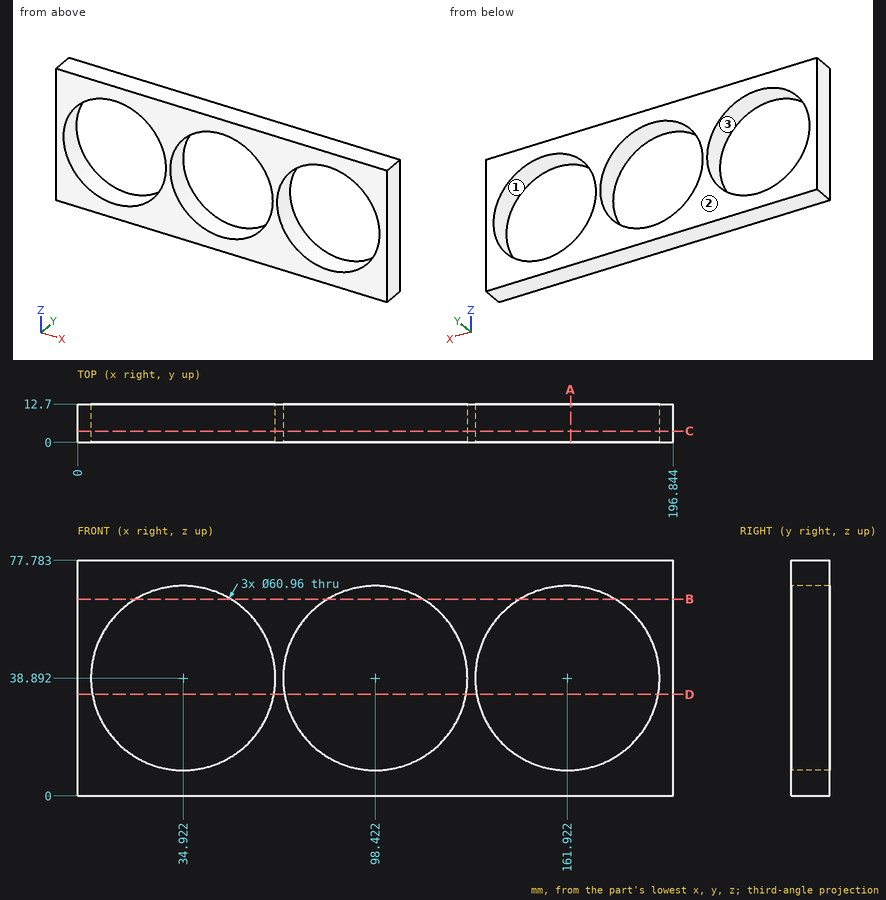
Answer from the drawing. Dimensions are ordinates in mm from the lowest x, y and z of the part. Give positions to 0.01 mm unless a question says otherwise; leave off trailing zeros. Write each loop counter-clockwise with the first axis right and the second up, starting at its lowest first coordinate (ties: lowest second). Pieces come first, ordered by that corner, then holes. Notation, with made-up numbers: M -5,53.5 L 49,53.5 A21 ccw 49,71.5 Z; hole C 56,36.25 d3. An arc over 180 degrees is marked long. Answer as CSV lines item,"result".
Q1. A cutting plane is placed at A-A on x = 163. Write down the section's boundary in (y, z), plus the area to 3 significant figures.
A:
outline,"M 0,0 L 12.7,0 L 12.7,8.43 L 0,8.43 Z; M 0,69.35 L 12.7,69.35 L 12.7,77.78 L 0,77.78 Z"
area,"214 mm²"
Q2. A cutting plane is placed at C-C on y = 3.75. Write down the section's boundary in (x, z) (1 decimal).
A:
outline,"M 0,0 L 196.8,0 L 196.8,77.8 L 0,77.8 Z; hole C 34.9,38.9 d61; hole C 98.4,38.9 d61; hole C 161.9,38.9 d61"
Q3. Find the intervals of material crossed by probe 1 along X at (y, z) = (2.25, 61.5) (1 decimal); probe 2 along X at (y, z) = (11.75, 44.5) (1 decimal); probe 3 along Z at (x, y) = (97.5, 9.25) (1 decimal), in increasing order. Write a range as [from, to].
A:
probe 1,"x = [0, 14.5], [55.4, 78], [118.9, 141.5], [182.4, 196.8]"
probe 2,"x = [0, 5], [64.9, 68.5], [128.4, 132], [191.9, 196.8]"
probe 3,"z = [0, 8.4], [69.4, 77.8]"
Q4. A cutting plane is placed at B-B on z = 65. Count the separate pieces of the cut face and the enclosed holes in it, plus the area to 3 significant figures.
A:
separate pieces,"4"
enclosed holes,"0"
area,"1,300 mm²"
Q5. The mould has two halves that part along X. Classify the marked faces 1, 2 and 3: +X half, -X half, draft (parallel to the pull), parting line (faces both ways), or undercut.
A:
face 1,"undercut"
face 2,"draft"
face 3,"undercut"
Q6. A cutting plane is placed at D-D on z = 33.5. Write down the section's boundary in (x, y) (1 decimal), plus the area to 3 significant figures.
A:
outline,"M 0,0 L 4.9,0 L 4.9,12.7 L 0,12.7 Z; M 64.9,0 L 68.4,0 L 68.4,12.7 L 64.9,12.7 Z; M 128.4,0 L 131.9,0 L 131.9,12.7 L 128.4,12.7 Z; M 191.9,0 L 196.8,0 L 196.8,12.7 L 191.9,12.7 Z"
area,"214 mm²"
